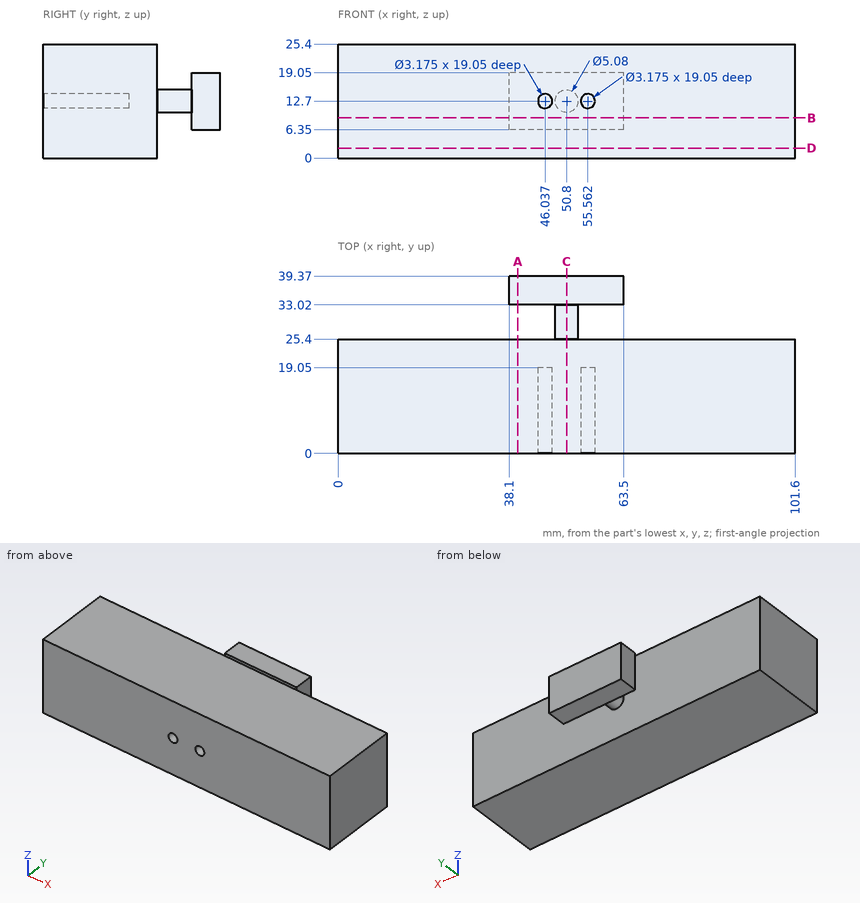
Check sheet for the drawn part. Datum: minimum x, y, z corner. Units: mm. Round coordinates to 2 decimals unless told otherwise and drop trailing zeros. Loops run counter-clockwise (first coordinate to the right, second up) from the corner with the lowest first, then second, coordinate; pieces in that order, holes last. Notation, with made-up numbers: (40.25, 87) - (59.25, 87) arc R24 ccw to (59.25, 97) - close; hole circle Ø1 at (54, -22.75). An arc over 180 degrees is marked (long way). Write item = value, one per line. Start each with the question number.
1. Section check B-B on z = 9. Enter the section's corners in (x, y).
2. Section check A-A on x = 40. Enter the section's corners in (y, z), then the cut area to 3 significant figures.
3. Thickness scan on line 1 (Y direction, x = 61, z = 12.25); line 2 (Y direction, x = 75, z = 8); line 3 (Z direction, x = 56.5, y = 18.5). Record the ranges inside material, lowest first.
4. Depth check by flat-ended pin: pin 1 (7 mm diameter, centred on x = 47.5, y = 37, fed in from -Z); pin 2 (10 mm diameter, centred on x = 10.5, z = 3.5, fed in from +Y); pin 3 (5 mm diameter, centred on y = 36, z = 13.5, fed in from +X). Enter the tip coordinate at first touch or a pass-through.
5. Section check C-C on x = 50.8. Enter the section's corners in (y, z).
6. Section check D-D on z = 2.25. Enter the section's corners in (x, y), then the cut area to 3 significant figures.
Working result:
q1.outline = (0, 0) - (101.6, 0) - (101.6, 25.4) - (0, 25.4) - close; (38.1, 33.02) - (63.5, 33.02) - (63.5, 39.37) - (38.1, 39.37) - close
q2.outline = (0, 0) - (25.4, 0) - (25.4, 25.4) - (0, 25.4) - close; (33.02, 6.35) - (39.37, 6.35) - (39.37, 19.05) - (33.02, 19.05) - close
q2.area = 726 mm^2
q3.line_1 = 0 to 25.4, 33.02 to 39.37
q3.line_2 = 0 to 25.4
q3.line_3 = 0 to 11.42, 13.98 to 25.4
q4.pin_1 = 6.35
q4.pin_2 = 25.4
q4.pin_3 = 63.5
q5.outline = (0, 0) - (25.4, 0) - (25.4, 10.16) - (33.02, 10.16) - (33.02, 6.35) - (39.37, 6.35) - (39.37, 19.05) - (33.02, 19.05) - (33.02, 15.24) - (25.4, 15.24) - (25.4, 25.4) - (0, 25.4) - close
q6.outline = (0, 0) - (101.6, 0) - (101.6, 25.4) - (0, 25.4) - close
q6.area = 2,580 mm^2
